CAD build for the part. Positions are in the model's coordinates, mm. A direction names the side the tool comes from. Round coordinates to 2 decimals unless told otherwise and drop trailing zeros. Loops run counter-clockwise (first coordinate to the right, second up) from the corner with the lowest first, then second, coordinate; pieces in that order, holes last. Notation, with made-up numbers: M 83,-23 L 135,-23 A30 cw 135,13 Z; hole C -7,-21.5 d5. An arc over 180 degrees is marked long. Use one line per item in the form item = value.
from build123d import *

# Parameters (mm, degrees)
SKETCH1_W           = 18.9
SKETCH1_H           = 6.35
SKETCH1_W_2         = 6.5
SKETCH1_H_2         = 4.35
BOSS_EXTRUDE1_DEPTH = 5
SKETCH2_W           = 18.9
SKETCH2_H           = 1
BOSS_EXTRUDE2_DEPTH = 10
SKETCH3_R           = 1.4
CUT_EXTRUDE1_DEPTH  = 2


with BuildPart() as part:
    # Sketch1 → Boss-Extrude1 (new body)
    with BuildSketch(Plane(origin=(0, 0, 0), x_dir=(1, 0, 0), z_dir=(0, 1, 0))):
        Rectangle(SKETCH1_W, SKETCH1_H)
        with Locations((-5.2, 0)):
            Rectangle(SKETCH1_W_2, SKETCH1_H_2, mode=Mode.SUBTRACT)
        with Locations((5.2, 0)):
            Rectangle(SKETCH1_W_2, SKETCH1_H_2, mode=Mode.SUBTRACT)
    extrude(amount=BOSS_EXTRUDE1_DEPTH)

    # Sketch2 → Boss-Extrude2 (add)
    with BuildSketch(Plane(origin=(0, 5, 0), x_dir=(1, 0, 0), z_dir=(0, 1, 0))):
        with Locations((0, 2.675)):
            Rectangle(SKETCH2_W, SKETCH2_H)
    extrude(amount=BOSS_EXTRUDE2_DEPTH)

    # Sketch3 → Cut-Extrude1 (cut, through all)
    with BuildSketch(Plane.XY.offset(-2.175)):
        with Locations((7.05, 12.6)):
            Circle(SKETCH3_R)
        with Locations((-7.05, 12.6)):
            Circle(SKETCH3_R)
    extrude(amount=-CUT_EXTRUDE1_DEPTH, mode=Mode.SUBTRACT)


solid = part.part
1. Cut at A-A on z = 1.5. Write the cut outline in (x, y).
Completed:
outline = M -9.45,0 L -8.45,0 L -8.45,5 L -9.45,5 Z; M -1.95,0 L 1.95,0 L 1.95,5 L -1.95,5 Z; M 8.45,0 L 9.45,0 L 9.45,5 L 8.45,5 Z
2. Cut at D-D on z = -2.5. Write the cut outline in (x, y), and give its area (3 significant figures).
Completed:
outline = M -9.45,0 L 9.45,0 L 9.45,15 L -9.45,15 Z; hole C -7.05,12.6 d2.8; hole C 7.05,12.6 d2.8
area = 271 mm2
3. Cut at B-B on x = -7.05. Write the cut outline in (y, z) (3 decimals), and give its area (3 significant figures).
Completed:
outline = M 0,-3.175 L 11.2,-3.175 L 11.2,-2.175 L 0,-2.175 Z; M 0,2.175 L 5,2.175 L 5,3.175 L 0,3.175 Z; M 14,-3.175 L 15,-3.175 L 15,-2.175 L 14,-2.175 Z
area = 17.2 mm2
4. Pull direction Y, two halves, no side cores. Call faces 1 (the face through (0, 0, 0)), 2 (the face through (0, 7, -2.175)), 3 (the face through (6.747, 11.233, -2.668)), 4 (the face through (0, 15, -3)): +Y half, -Y half, draft (parallel to the pull), parting line (faces both ways), or undercut.
Completed:
face_1 = -Y half
face_2 = draft
face_3 = undercut
face_4 = +Y half
5. Cut at C-C on y = 3.5. Write the cut outline in (x, z) (3 decimals), and give its area (3 significant figures).
Completed:
outline = M -9.45,-3.175 L 9.45,-3.175 L 9.45,3.175 L -9.45,3.175 Z; hole M -8.45,-2.175 L -1.95,-2.175 L -1.95,2.175 L -8.45,2.175 Z; hole M 1.95,-2.175 L 8.45,-2.175 L 8.45,2.175 L 1.95,2.175 Z
area = 63.5 mm2
6. Drop flat-ended pins along their axis: P1, Ø1.7, axis at x = 7.05, y = 12.6, coming from the +Z side; P2, Ø2, axis at x = 7, y = 10, coming from the +Z side (3 decimals). Give the stop position or say it passes through.
Completed:
P1 = through
P2 = -2.175
7. Tool access for faces 5 (the face through (8.45, 2, 0)), 6 (the face through (-6.4, 11.36, -2.67)), 7 (the face through (-2, 5, 3)): list every direction of +Z, -Z, +X, -X, +Y, -Y with a clear straight run to the whole face (end or side of a thin tool).
Completed:
face_5 = +Y, -Y
face_6 = +Z, -Z
face_7 = +Z, +X, -X, +Y
8. Probe line 1 along Z through (x, y) = (5, 2.5) (3 decimals); line 2 along X through (y, z) = (3, -1); line 3 along Y through (x, z) = (-7.05, -2.5). List the from-to ranges inside material, lowest first. Write a range as from..to.
Completed:
line_1 = -3.175..-2.175, 2.175..3.175
line_2 = -9.45..-8.45, -1.95..1.95, 8.45..9.45
line_3 = 0..11.2, 14..15
